Geometry: final body of the model. Coordinates: model frame, mm. Round coordinates to 2 decimals unless told otherwise and drop trailing zeros. Loops run counter-clockwise (first coordinate to the right, second up) from the corner with the lowest first, then second, coordinate; pieces in that order, holes last. Notation, with made-up numbers: (4.25, 61) - (54.25, 61) arc R23 ccw to (54.25, 79) - close; hole circle Ø1 at (42, 6). An arc over 180 degrees is marked (long way). Use CSV: the item, a comma, the result in double quotes.
from build123d import *

# Parameters (mm, degrees)
BOSS_EXTRUDE1_DEPTH = 81.6
FILLET1_R           = 5.5


with BuildPart() as part:
    # Sketch1 → Boss-Extrude1 (new body)
    with BuildSketch(Plane(origin=(0, 0, 0), x_dir=(0, 0, -1), z_dir=(1, 0, 0))):
        Polygon((-27.320490368, 28.152364273), (22.679509632, 28.152364273), (22.679509632, -31.847635727), (-12.951148339, -31.847635727), (-27.320490368, 15.152364273), align=None)
    extrude(amount=BOSS_EXTRUDE1_DEPTH)

    # Fillet1
    fillet1_edges = [part.edges().sort_by_distance(p)[0] for p in [
        (40.8, 28.152364273, 27.320490368),
        (40.8, 28.152364273, -22.679509632),
        (40.8, -31.847635727, -22.679509632),
        (40.8, -31.847635727, 12.951148339),
    ]]
    fillet(fillet1_edges, radius=FILLET1_R)


solid = part.part
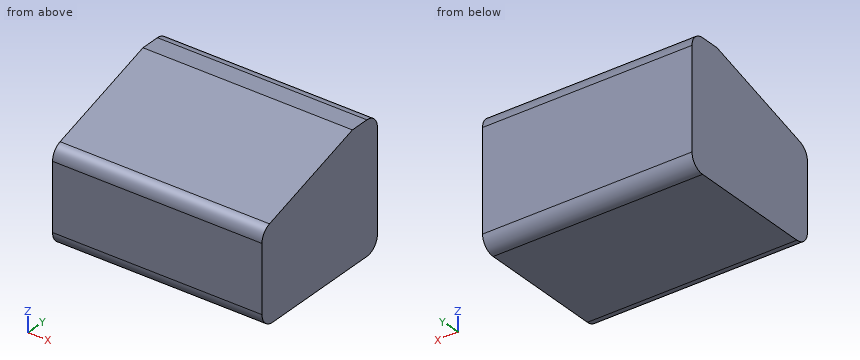
Item 1: Section C-C on y = -9. Return the cut outline in (x, z).
Final values:
outline,"(0, -22.68) - (81.6, -22.68) - (81.6, 19.94) - (0, 19.94) - close"
Item 2: Section B-B on y = -18.5. Return the cut outline in (x, z).
Final values:
outline,"(0, -22.68) - (81.6, -22.68) - (81.6, 17.03) - (0, 17.03) - close"
Item 3: Section A-A on x = 34.5. Return the cut outline in (y, z).
Final values:
outline,"(-31.85, -17.18) arc R5.5 ccw to (-26.35, -22.68) - (22.65, -22.68) arc R5.5 ccw to (28.15, -17.18) - (28.15, 21.82) arc R5.5 ccw to (22.65, 27.32) - (15.15, 27.32) - (-27.96, 14.14) arc R5.5 ccw to (-31.85, 8.88) - close"
Item 4: Pin query (flat end, axial travel): P1, Ø12, axis at y = -14.5, z = -17.5, coming from the -X side; P2, Ø8, axis at x = 63, z = 14, coming from the -Y side. Return the tip coordinate at first contact, or that it passes through.
Final values:
P1,"stops at x = 0"
P2,"stops at y = -31.73"
Item 5: Material intervals for line 1 (Z direction, x = 77, y = 14.5); line 2 (Y direction, x = 45.5, z = -20); line 3 (Y direction, x = 17, z = -19.5), sorted ascending.
Final values:
line 1,"z = -22.68 to 27.12"
line 2,"y = -31.07 to 27.37"
line 3,"y = -31.33 to 27.64"
